Autodesk Inventor part; units mm, degrees
ref_plane "Work Plane1" through (0, 15, 0) normal (0, 1, 0) x (-1, 0, 0)
ref_plane "YZ Plane" through (0, 0, 0) normal (1, 0, 0) x (0, 1, 0)
ref_plane "XY Plane" through (0, 0, 0) normal (0, 0, 1) x (1, 0, 0)
sketch "Sketch1" plane through (0, 0, 0) normal (0, 0, 1) x (1, 0, 0)
  line L0 (0, 0) -> (0, 20)
  line L1 (0, 0) -> (20, 0)
  arc A0 (20, 0) -> (0, 20) centre (0, 0) ccw
  line L2 (0, -4.8284) -> (0, 28.9706)
  dimension "d2" = 20
revolve "Revolution1" add sketch "Sketch1" angle 360 about axis through (0, -10, 0) along (0, 1, 0)
ref_plane "Work Plane1" through (0, 15, 0) normal (0, 1, 0) x (-1, 0, 0)
sketch "Sketch2" plane through (0, 15, 0) normal (0, 1, 0) x (-1, 0, 0)
  point P0 (0, 0)
  point P1 (0, 0)
hole "Hole1" at (0, 15, 0) direction (0, -1, 0) diameter 4.5 end through all counterbore diameter 8 counterbore depth 4
shell "Shell1" thickness 6 removed faces 1 at (13.8841, 0, 1.6858)
sketch "Sketch3" plane through (0, 0, 0) normal (0, -1, 0) x (1, 0, 0)
  circle A0 centre (0, 0) radius 8.25
  circle A1 centre (0, 0) radius 2.25
extrude "Extrusion1" cut sketch "Sketch3" against normal blind 5
properties part number "Ball_Upper Half" material "Nylon 6/6"
The listing builds one solid part. Answer for the finished solid, in the listing's coordinates (mm). A direction names the side the tool comes from. Round coordinates to 2 decimals unless told otherwise and drop trailing zeros. Loops run counter-clockwise (first coordinate to the right, second up) from the corner with the lowest first, then second, coordinate; pieces in that order, holes last.
Q1. Given pin 1 Ø1 at (x, y) = (13.5, 17.5) entering from -Z; pin 2 Ø5 at (x, y) = (10, 10.5) entering from -Z; pin 3 Ø9 at (x, z) = (0, 0) entering from -Y; pin 4 Ø10 at (x, y) = (1, 18) entering from -Z, each flat-ended and moving along its own axis, determine where each tip first touches the part or whether it passes through.
Q2. Section A-A, the plane x = 0 is taken. Determine the outline of the cut face in (y, z), then the cut area to 3 significant figures.
Q3. Section B-B, the plane z = 0 is taken. Determine the outline of the cut face in (x, y).
Q4. Section C-C, the plane y = 14.25 is taken. Determine the outline of the cut face in (x, z).
Q5. For a pull along Z with two mould halves and no side action, classify faces 3 (the face through (2, 11, 2)), 4 (the face through (-4, 0, -14)) as released by +Z, released by -Z, zero draft, split by the parting line, or undercut.
Q6. Find the intervals of material crossed by line 1 (X direction, y = 6.75, z = -3.5); line 2 (Z direction, x = -0.5, y = 9.5); line 3 (Z direction, x = 0, y = 12.55), in increasing order.
Q7. Which of the six approach directions +Z, -Z, +X, -X, +Y, -Y give full straight-line access (tool end or side, diameter ignored) to faces 1 (the face through (0, 15, 0)), 2 (the face through (-2.23, 7.96, -0.29))?
Q8. Section D-D, the plane x = -4.5 is taken. Determine the outline of the cut face in (y, z), then the cut area to 3 significant figures.
Completed:
1. pin 1: passes through
1. pin 2: stops at z = -16
1. pin 3: stops at y = 5
1. pin 4: stops at z = -15.17
2. outline: (0, -20) arc R20 ccw to (0, 20) - (0, 14) arc R14 cw to (9.8, 10) - (5, 10) - (5, 2.25) - (11, 2.25) - (11, 4) - (15, 4) - (15, -4) - (11, -4) - (11, -2.25) - (5, -2.25) - (5, -10) - (9.8, -10) arc R14 cw to (0, -14) - close
2. area: 415 mm2
3. outline: (-20, 0) - (-14, 0) arc R14 cw to (-10, 9.8) - (-10, 5) - (-2.25, 5) - (-2.25, 11) - (-4, 11) - (-4, 15) - (4, 15) - (4, 11) - (2.25, 11) - (2.25, 5) - (10, 5) - (10, 9.8) arc R14 cw to (14, 0) - (20, 0) arc R20 ccw to start
4. outline: circle Ø28.07 at (0, 0); hole circle Ø8 at (0, 0)
5. face 3: undercut
5. face 4: zero draft
6. line 1: x = -18.5 to -11.76, -9.37 to 9.37, 11.76 to 18.5
6. line 2: z = -17.59 to -10.27, -9.99 to -2.19, 2.19 to 9.99, 10.27 to 17.59
6. line 3: z = -15.57 to -4, 4 to 15.57
7. face 1: none
7. face 2: -Y
8. outline: (0, -19.49) arc R19.49 ccw to (0, 19.49) - (0, 13.26) arc R13.26 cw to (9.8, 8.93) - (5, 8.93) - (5, -8.93) - (9.8, -8.93) arc R13.26 cw to (0, -13.26) - close
8. area: 449 mm2
